Can you work these out from the model? Positions are in its coordinate system, mm. Face numbers are marked on the shaded views. Give positions to 0.01 mm unless a question says otherwise; leave off trailing zeros. Order: outer loops, then holes, each group sorted by start corner. A loop starts at its lowest first (then second) coordinate and runs counter-clockwise, first axis right, second up. Notation, with made-up numbers: (58.5, 53.25) - (80.5, 53.25) arc R12 cw to (80.5, 72.25) - close; hole circle Ø9 at (39.5, 28.25). An arc over 180 degrees is marked (long way). Return JSON: item names as keys, results as strings.
```python
from build123d import *

# Parameters (mm, degrees)
F1_DEPTH = 168


# Not quite as in the source:
# - a feature names something its author has since deleted; it is built from what else it names


with BuildPart() as f1:
    # F0 (on Top) → F1 (new body)
    with BuildSketch(Plane.XY):
        with BuildLine():
            add(Edge.make_bspline(
                [(9.0589725163, 14.9090803276), (9.1893761129, 14.9089854783), (9.3201289556, 14.9089586218), (9.4512325362, 14.909)],
                knots=[108.3727376298, 108.3727376298, 108.3727376298, 108.3727376298, 108.6044995707, 108.6044995707, 108.6044995707, 108.6044995707], degree=3))
            ThreePointArc((9.0589725163, 14.9090803276), (-12.3350874174, 11.9828700727), (-32.1953748348, 3.5071700662))
            Line((-32.1953748348, 3.5071700662), (-32.1954637008, 6.33471e-05))
            Line((-32.1954637008, 6.33471e-05), (-32.1955525689, -3.5071262621))
            ThreePointArc((-32.1955525689, -3.5071262621), (-12.3352527385, -11.9828512354), (9.0588260182, -14.9090804342))
            add(Edge.make_bspline(
                [(9.0588260182, -14.9090804342), (9.1892781859, -14.9089854984), (9.3200798608, -14.9089586063), (9.4512325362, -14.909)],
                knots=[108.372650841, 108.372650841, 108.372650841, 108.372650841, 108.6044995707, 108.6044995707, 108.6044995707, 108.6044995707], degree=3))
            Line((9.4512325362, -14.909), (13.4156349212, -15.0296401869))
            ThreePointArc((13.4156349212, -15.0296401869), (26.4575983511, -11.3147653424), (33.9237386916, 0.0055638769))
            ThreePointArc((33.9237386916, 0.0055638769), (26.221744338, 11.4277863656), (12.8924894738, 14.909))
            Line((12.8924894738, 14.909), (9.4512325362, 14.909))
        make_face()
        with BuildLine():
            Line((-29.6955161871, -2.0713442572), (-29.6954637016, 0))
            Line((-29.6954637016, 0), (-29.6954112161, 2.0713449993))
            ThreePointArc((-29.6954112161, 2.0713449993), (-11.0041823718, 9.7538427825), (9.0291136139, 12.409))
            Line((9.0291136139, 12.409), (13.0291136139, 12.409))
            ThreePointArc((13.0291136139, 12.409), (24.4821941123, 9.5918072896), (31.3456378974, 0))
            ThreePointArc((31.3456378974, 0), (24.7175372439, -9.4867852182), (13.5527042793, -12.5326540468))
            Line((13.5527042793, -12.5326540468), (4.2194331318, -12.2486345488))
            ThreePointArc((4.2194331318, -12.2486345488), (-13.3194868099, -9.0976060688), (-29.6955161871, -2.0713442572))
        make_face(mode=Mode.SUBTRACT)
    extrude(amount=-F1_DEPTH)


solid = f1.part
```
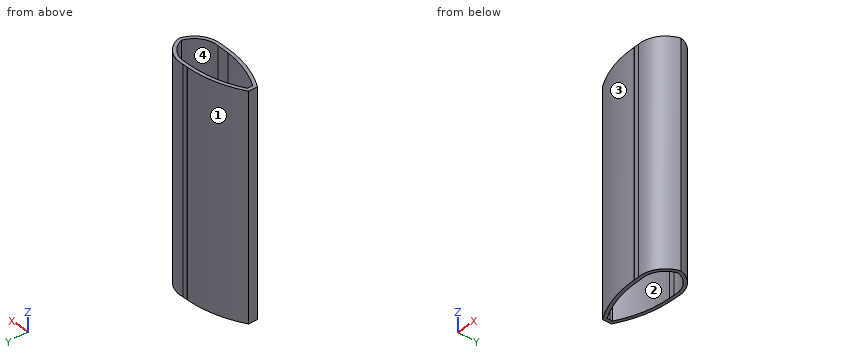
1. For pin 1 Ø6 at (y, z) = (6, -117) entering from +X; pin 2 Ø10 at (y, z) = (2.5, -43) entering from +X; pin 3 Ø5 at (y, z) = (11.5, -30.5) entering from +X, each with a flat end and sliding along its axis, tell me the tip position at first contact or that it passes through.
Checks:
{"pin 1": "x = 32.95", "pin 2": "x = 33.92", "pin 3": "x = 29.04"}
2. Thinking about a two-plate mould opening in Y: for the marked faces 1, 2, 3 and 4, which applies, +Y half, -Y half, draft (parallel to the pull), parting line (faces both ways), or undercut?
Checks:
{"face 1": "+Y half", "face 2": "undercut", "face 3": "-Y half", "face 4": "undercut"}
3. Suppose I cut it at B-B (y = -6.5). List the corners of the cut face in (x, z) for me, plus the area to 3 significant figures.
Checks:
{"outline": "(-26.7, -168) - (-20.64, -168) - (-20.64, 0) - (-26.7, 0) - close; (27.96, -168) - (31.09, -168) - (31.09, 0) - (27.96, 0) - close", "area": "1,540 mm^2"}
4. Suppose I cut it at A-A (x = -12.5). List the corners of the cut face in (y, z) for me.
Checks:
{"outline": "(-11.94, -168) - (-9.34, -168) - (-9.34, 0) - (-11.94, 0) - close; (9.34, -168) - (11.94, -168) - (11.94, 0) - (9.34, 0) - close"}
5. If I drill on L1, parallel to Y at x = 9, z = -137; L2, parallel to Y at x = 0.5, z = -79; L3, parallel to X at y = 5, z = -151, over which ranges is the centre line in solid material (lowest first)? Write a range as [from, to].
Checks:
{"L1": "[-14.91, -12.39], [12.41, 14.91]", "L2": "[-14.44, -11.92], [11.92, 14.44]", "L3": "[-29.58, -24.05], [29.06, 31.99]"}
